Geometry check sheet. Reference: the model listing, model coordinates, mm. A direction names the side the tool comes from. Coordinates: 2 decimals unless noted, no trailing zeros. Order: outer loops, then holes, each group sorted by start corner. A loop starts at its lowest first (then second) coordinate and runs counter-clockwise, first axis right, second up. Notation, with made-up numbers: (68, 3) - (92, 3) arc R23 ccw to (92, 36) - close; hole circle Ø9 at (41, 60). An arc over 180 degrees is marked (long way). Use CSV: the item, a comma, the result in double quotes. Start each with the question number.
1) Sectioned sample at C-C, the plane y = 21. Record the cut outline in (x, z), and give its area (3 significant figures).
2) Depth check by flat-ended pin: P1, Ø16, axis at x = 125, y = 11.5, coming from the -Z side; P2, Ø7.5, axis at y = -11, z = -3, coming from the +X side; P3, Ø14.5, axis at x = 125.5, y = 21, coming from the -Z side. Enter the tip coordinate at first touch or a pass-through.
3) Thickness scan on probe 1 along Y at (x, z) = (125, -1); probe 2 along X at (y, z) = (26, -18); probe 3 along Y at (x, z) = (27.5, -17). Record the ranges inside material, lowest first. Write a range as [from, to].
4) Sectioned sample at B-B, the plane y = 30. Record the cut outline in (x, z), and give its area (3 significant figures).
5) Sectioned sample at D-D, the plane z = -5.5. Record the cut outline in (x, y), and give its area (3 significant figures).
6) Tool access check on faces 5 (the cylindrical face through (9.165, 6.949, -38.025)), 6 (the flat face through (99.15, 12, -76)), 7 (the flat face through (56, -2, -7)), 8 (the flat face through (69.5, -10, -3)). Record the directions out of +Z, -Z, +X, -X, +Y, -Y that give a thin tool (end or side, any length) a straight path to the whole face; none if there is none.
7) Draft check along Z on faces 1 (the cylindrical face through (109.051, 7.165, -25.35)), 2 (the flat face through (113, 13, -50)), 3 (the flat face through (116, 9, -24)), 4 (the flat face through (117.7, 6.4, -16)). Enter one of: released by +Z, released by -Z, zero draft, split by the parting line, or undercut.
8) Sectioned sample at A-A, the plane x = 125.5. Record the cut outline in (y, z).
from build123d import *

# Parameters (mm, degrees)
ESQUISSE1_W             = 138
ESQUISSE1_H             = 75
BOSS_EXTRU_1_DEPTH      = 3
ESQUISSE2_W             = 5
ESQUISSE2_H             = 75
ESQUISSE2_W_2           = 25
BOSS_EXTRU_2_DEPTH      = 30
CONG_1_R                = 13.85
ESQUISSE3_W             = 138
ESQUISSE3_H             = 33
BOSS_EXTRU_3_DEPTH      = 5
ESQUISSE5_W             = 20
ESQUISSE5_H             = 76
ENL_V_MAT_EXTRU_2_DEPTH = 30
ESQUISSE6_R             = 6.25
ENL_V_MAT_EXTRU_3_DEPTH = 4
ESQUISSE7_W             = 20
ESQUISSE7_H             = 3
ENL_V_MAT_EXTRU_4_DEPTH = 30
ENL_V_MAT_EXTRU_5_REACH = 164.89
ESQUISSE8_W             = 18.85
ESQUISSE8_H             = 30
ESQUISSE10_W            = 8
ESQUISSE10_H            = 15
ENL_V_MAT_EXTRU_6_DEPTH = 3
ENL_V_MAT_EXTRU_7_DEPTH = 3
ESQUISSE12_W            = 80
ESQUISSE12_H            = 33
ENL_V_MAT_EXTRU_8_DEPTH = 2
BOSS_EXTRU_4_DEPTH      = 7
ESQUISSE14_W            = 23
ESQUISSE14_H            = 14.5
ENL_V_MAT_EXTRU_9_DEPTH = 7
CONG_2_R                = 10


with BuildPart() as part:
    # Esquisse1 → Boss.-Extru.1 (new body)
    with BuildSketch(Plane(origin=(0, 0, 0), x_dir=(1, 0, 0), z_dir=(0, 1, 0))):
        with Locations((69, 37.5)):
            Rectangle(ESQUISSE1_W, ESQUISSE1_H)
    extrude(amount=BOSS_EXTRU_1_DEPTH)

    # Esquisse2 → Boss.-Extru.2 (add)
    with BuildSketch(Plane(origin=(0, 3, 0), x_dir=(1, 0, 0), z_dir=(0, 1, 0))):
        with Locations((2.5, 37.5)):
            Rectangle(ESQUISSE2_W, ESQUISSE2_H)
        with Locations((125.5, 37.5)):
            Rectangle(ESQUISSE2_W_2, ESQUISSE2_H)
    extrude(amount=BOSS_EXTRU_2_DEPTH)

    # Congé1
    cong_1_edges = [part.edges().sort_by_distance(p)[0] for p in [
        (5, 3, -37.5),
        (113, 3, -37.5),
    ]]
    fillet(cong_1_edges, radius=CONG_1_R)

    # Esquisse3 → Boss.-Extru.3 (add)
    with BuildSketch(Plane(origin=(0, 0, -75), x_dir=(-1, 0, 0), z_dir=(0, 0, -1))):
        with Locations((-69, 16.5)):
            Rectangle(ESQUISSE3_W, ESQUISSE3_H)
    extrude(amount=BOSS_EXTRU_3_DEPTH)

    # Esquisse5 → Enlèv. mat.-Extru.2 (cut)
    with BuildSketch(Plane(origin=(0, 33, 0), x_dir=(1, 0, 0), z_dir=(0, 1, 0))):
        with Locations((128, 42)):
            Rectangle(ESQUISSE5_W, ESQUISSE5_H)
    extrude(amount=-ENL_V_MAT_EXTRU_2_DEPTH, mode=Mode.SUBTRACT)

    # Esquisse6 → Enlèv. mat.-Extru.3 (cut)
    with BuildSketch(Plane.XY):
        with Locations((125.5, 21)):
            Circle(ESQUISSE6_R)
    extrude(amount=-ENL_V_MAT_EXTRU_3_DEPTH, mode=Mode.SUBTRACT)

    # Esquisse7 → Enlèv. mat.-Extru.4 (cut)
    with BuildSketch(Plane(origin=(0, 0, -80), x_dir=(-1, 0, 0), z_dir=(0, 0, -1))):
        with Locations((-128, 1.5)):
            Rectangle(ESQUISSE7_W, ESQUISSE7_H)
    extrude(amount=-ENL_V_MAT_EXTRU_4_DEPTH, mode=Mode.SUBTRACT)

    # Enlèv. mat.-Extru.5: up to this face of the body (flat: up to its plane)
    enl_v_mat_extru_5_end = Plane(part.part.faces().sort_by_distance((65.609195402, 0, -38.563218391))[0])
    # Esquisse8 → Enlèv. mat.-Extru.5 (cut, up to the picked face)
    with BuildSketch(Plane(origin=(0, 33, 0), x_dir=(1, 0, 0), z_dir=(0, 1, 0)), mode=Mode.PRIVATE) as enl_v_mat_extru_5_sk1:
        with Locations((108.575, 65)):
            Rectangle(ESQUISSE8_W, ESQUISSE8_H)
    enl_v_mat_extru_5_tool1 = split(extrude(enl_v_mat_extru_5_sk1.sketch, amount=-ENL_V_MAT_EXTRU_5_REACH, mode=Mode.PRIVATE), bisect_by=enl_v_mat_extru_5_end, keep=Keep.BOTH, mode=Mode.PRIVATE)
    add(enl_v_mat_extru_5_tool1.solids().sort_by(Axis((108.575, 33, -65), (0, -1, 0)))[0], mode=Mode.SUBTRACT)

    # Esquisse10 → Enlèv. mat.-Extru.6 (cut)
    with BuildSketch(Plane(origin=(118, 0, 0), x_dir=(0, 0, -1), z_dir=(1, 0, 0))):
        with Locations((20, 10.5)):
            Rectangle(ESQUISSE10_W, ESQUISSE10_H)
    extrude(amount=-ENL_V_MAT_EXTRU_6_DEPTH, mode=Mode.SUBTRACT)

    # Esquisse11 → Enlèv. mat.-Extru.7 (cut)
    with BuildSketch(Plane(origin=(0, 3, 0), x_dir=(1, 0, 0), z_dir=(0, 1, 0))):
        Polygon((115, 24), (118, 24), (118, 50), (138, 50), (138, 4), (131, 4), (131, 16), (115, 16), align=None)
    extrude(amount=-ENL_V_MAT_EXTRU_7_DEPTH, mode=Mode.SUBTRACT)

    # Esquisse12 → Enlèv. mat.-Extru.8 (cut)
    with BuildSketch(Plane.ZY):
        with Locations((-40, 16.5)):
            Rectangle(ESQUISSE12_W, ESQUISSE12_H)
    extrude(amount=-ENL_V_MAT_EXTRU_8_DEPTH, mode=Mode.SUBTRACT)

    # Esquisse13 → Boss.-Extru.4 (add)
    with BuildSketch(Plane.XY):
        Polygon((37, 0), (44.596875763, -20), (71.596875763, -20), (78, 0), align=None)
    extrude(amount=-BOSS_EXTRU_4_DEPTH)

    # Esquisse14 → Enlèv. mat.-Extru.9 (cut)
    with BuildSketch(Plane.XY):
        with Locations((58, -9.75)):
            Rectangle(ESQUISSE14_W, ESQUISSE14_H)
    extrude(amount=-ENL_V_MAT_EXTRU_9_DEPTH, mode=Mode.SUBTRACT)

    # Congé2
    cong_2_edges = [part.edges().sort_by_distance(p)[0] for p in [
        (37, 0, -3.5),
        (78, 0, -3.5),
        (124.5, 3, -4),
    ]]
    fillet(cong_2_edges, radius=CONG_2_R)


solid = part.part
Evaluation:
1,outline,"(2, -80) - (99.15, -80) - (99.15, -75) - (5, -75) - (5, 0) - (2, 0) - close; (113, -50) - (118, -50) - (118, -4) - (119.25, -4) - (119.25, 0) - (113, 0) - close; (131.75, -4) - (138, -4) - (138, 0) - (131.75, 0) - close"
1,area,"991 mm²"
2,P1,"z = -50"
2,P2,"x = 75.68"
2,P3,"z = -4"
3,probe 1,"[0, 14.77], [27.23, 33]"
3,probe 2,"[2, 5], [113, 118]"
3,probe 3,"[0, 3]"
4,outline,"(2, -80) - (99.15, -80) - (99.15, -75) - (5, -75) - (5, 0) - (2, 0) - close; (113, -50) - (118, -50) - (118, -4) - (138, -4) - (138, 0) - (113, 0) - close"
4,area,"1,040 mm²"
5,outline,"(2, 0) - (30.1, 0) arc R10 cw to (39.45, -6.45) - (44.6, -20) - (71.6, -20) - (75.77, -6.95) arc R10 cw to (85.3, 0) - (131, 0) - (131, 7.73) - (118, 7.73) - (118, 33) - (113, 33) - (113, 16.85) arc R13.85 cw to (99.15, 3) - (18.85, 3) arc R13.85 cw to (5, 16.85) - (5, 33) - (2, 33) - close; hole (46.5, -17) - (69.5, -17) - (69.5, -2.5) - (46.5, -2.5) - close"
5,area,"1,140 mm²"
6,face 5,"+Z, +Y"
6,face 6,"-Z, +X, +Y, -Y"
6,face 7,"-Z, +X, -X, -Y"
6,face 8,"+Z, -Z"
7,face 1,"zero draft"
7,face 2,"released by -Z"
7,face 3,"undercut"
7,face 4,"undercut"
8,outline,"(0, -16) - (3, -16) - (3, -14) arc R10 cw to (13, -4) - (14.75, -4) - (14.75, 0) - (0, 0) - close; (27.25, -4) - (33, -4) - (33, 0) - (27.25, 0) - close"
